Autodesk Inventor part; units mm, degrees
ref_plane "YZ Plane" through (0, 0, 0) normal (1, 0, 0) x (0, 1, 0)
ref_plane "XZ Plane" through (0, 0, 0) normal (0, 1, 0) x (-1, 0, 0)
ref_plane "XY Plane" through (0, 0, 0) normal (0, 0, 1) x (1, 0, 0)
sketch "Sketch1" plane through (0, 0, 0) normal (0, 0, 1) x (1, 0, 0)
  line L0 (0, 0) -> (25.4, 0)
  line L1 (25.4, 0) -> (25.4, 25.4)
  line L2 (25.4, 25.4) -> (0, 25.4)
  line L3 (0, 25.4) -> (0, 0)
  line L4 (1.5875, 23.8125) -> (23.8125, 23.8125)
  line L5 (23.8125, 23.8125) -> (23.8125, 1.5875)
  line L6 (23.8125, 1.5875) -> (1.5875, 1.5875)
  line L7 (1.5875, 1.5875) -> (1.5875, 23.8125)
  dimension "d0" = 25.4
  dimension "d1" = 25.4
  dimension "d4" = 1.5875
extrude "Extrusion1" add sketch "Sketch1" against normal blind 25.4 contours L3 L2 L1 L0 | L4 L5 L6 L7
extrude "Extrusion2" add sketch "Sketch1" along normal blind 25.4 contours L4 L5 L6 L7
sketch "Sketch2" plane through (25.4, 0, 0) normal (1, 0, 0) x (0, 0, -1)
  line L0 (25.4, 0) -> (25.4, 25.4)
  line L1 (0, 25.4) -> (25.4, 25.4)
  line L2 (0, 0) -> (0, 25.4)
  line L3 (0, 0) -> (25.4, 0)
  line L4 (23.8125, 23.8125) -> (23.8125, 1.5875)
  line L5 (23.8125, 1.5875) -> (1.5875, 1.5875)
  line L6 (1.5875, 1.5875) -> (1.5875, 23.8125)
  line L7 (1.5875, 23.8125) -> (23.8125, 23.8125)
  dimension "d8" = 1.5875
sketch "Sketch3" plane through (0, 25.4, 0) normal (0, 1, 0) x (1, 0, 0)
  line L0 (25.4, 25.4) -> (0, 25.4)
  line L1 (0, 0) -> (0, 25.4)
  line L2 (25.4, 0) -> (0, 0)
  line L3 (25.4, 0) -> (25.4, 25.4)
  line L4 (1.5875, 23.8125) -> (23.8125, 23.8125)
  line L5 (23.8125, 23.8125) -> (23.8125, 1.5875)
  line L6 (23.8125, 1.5875) -> (1.5875, 1.5875)
  line L7 (1.5875, 1.5875) -> (1.5875, 23.8125)
  dimension "d9" = 1.5875
extrude "Extrusion3" add sketch "Sketch2" along normal blind 25.4 contours L4 L5 L6 L7
extrude "Extrusion4" add sketch "Sketch3" along normal blind 25.4 contours L4 L5 L6 L7
sketch "Sketch4" plane through (1.5875, 25.4, -23.8125) normal (-1, 0, 0) x (0, 0, 1)
  point P0 (23.8125, -25.4)
  point P1 (11.1125, 12.7)
hole "Hole1" at (1.5875, 38.1, -12.7) direction (1, 0, 0) diameter 6.35 depth 25.4 tip angle 118
sketch "Sketch5" plane through (23.8125, 25.4, -23.8125) normal (0, 0, -1) x (-1, 0, 0)
  point P0 (23.8125, -25.4)
  point P1 (11.1125, 12.7)
hole "Hole2" at (12.7, 38.1, -23.8125) direction (0, 0, 1) diameter 6.35 depth 25.4 tip angle 118
sketch "Sketch6" plane through (1.5875, 23.8125, 25.4) normal (0, 1, 0) x (1, 0, 0)
  line L0 (0, 25.4) -> (22.225, 25.4)
  line L1 (23.8125, 25.4) -> (23.8125, 50.8)
  point P0 (-1.5875, 25.4)
  point P1 (11.1125, 12.7)
  point P2 (36.5125, 38.1)
  dimension "d28" = 12.7
  dimension "d29" = 12.7
hole "Hole3" at (12.7, 23.8125, 12.7) at (38.1, 23.8125, -12.7) direction (0, -1, 0) diameter 6.35 depth 25.4 tip angle 118
properties part number "3-way corner"
Model file for the job. Use its own axes, mm. A direction names the side the tool comes from. Coordinates: 2 decimals unless noted, no trailing zeros. Order: outer loops, then holes, each group sorted by start corner. A loop starts at its lowest first (then second) coordinate and runs counter-clockwise, first axis right, second up. Notation, with made-up numbers: M -9.75,-25 L 30.25,-25 A22 cw 30.25,-18 Z; hole C 62.5,18 d8. An arc over 180 degrees is marked long. Answer as CSV lines item,"result".
(1) Band-saw the part on C-C, the plane x = 38.1. List the corners of the cut face in (y, z) (1 decimal), then the cut area to 3 significant figures.
Geometry says:
outline,"M 1.6,-23.8 L 23.8,-23.8 L 23.8,-15.9 L 1.6,-15.9 Z; M 1.6,-9.5 L 23.8,-9.5 L 23.8,-1.6 L 1.6,-1.6 Z"
area,"353 mm2"
(2) 3-axis set-ups, long thin cutter, end or side, ignore diameter. For faces 5 (the flat face through (35, 23.812, -10)), 6 (the flat face through (1.588, 13, 13)), 7 (the flat face through (10, 23.812, 15)), 8 (the flat face through (23.812, 13, 13)): which of +Z, -Z, +X, -X, +Y, -Y reach the whole face in a straight line?
Geometry says:
face 5,"+Z, -Z, +X, +Y"
face 6,"+Z, -X, +Y, -Y"
face 7,"+Z, +X, -X, +Y"
face 8,"+Z, +X, +Y, -Y"
(3) Flat gauge pins, fed straight in: pin 1 (6.5 mm diameter, centred on x = 42.5, y = 7.5, fed in from -Z); pin 2 (12 mm diameter, centred on x = 23, y = 33, fed in from +Z); pin 3 (18 mm diameter, centred on x = 35.5, z = -9, fed in from -Y). Where does each tip first touch, or does it go through?
Geometry says:
pin 1,"stops at z = -23.81"
pin 2,"stops at z = -1.59"
pin 3,"stops at y = 1.59"
(4) Pull direction Y, two halves, no side cores. Call faces 1 (the cylindrical face through (13.92, 41.03, -19.41)), 2 (the cylindrical face through (5.987, 35.423, -10.993)), 3 (the flat face through (1.588, 35, -10)), 4 (the flat face through (13, 0, -13)): +Y half, -Y half, draft (parallel to the pull), parting line (faces both ways), or undercut.
Geometry says:
face 1,"undercut"
face 2,"undercut"
face 3,"draft"
face 4,"-Y half"
(5) Band-saw the part on D-D, the plane z = -14.5. State how many separate pieces and enclosed holes the cut face has, then the cut area to 3 significant figures.
Geometry says:
separate pieces,"3"
enclosed holes,"0"
area,"1,540 mm2"
(6) Band-saw the part on B-B, the plane z = 12.7. List the corners of the cut face in (x, y) (1 decimal).
Geometry says:
outline,"M 1.6,1.6 L 9.5,1.6 L 9.5,23.8 L 1.6,23.8 Z; M 15.9,1.6 L 23.8,1.6 L 23.8,23.8 L 15.9,23.8 Z"
(7) Wall check: line 1 along Z through (x, y) = (12.7, 8.5) (3 decimals); line 2 along Y through (x, z) = (12.7, -17.5) (3 decimals); line 3 along X through (y, z) = (38, -17). Give the ranges that are in metal, low to high.
Geometry says:
line 1,"z = -25.4 to 9.525, 15.875 to 25.4"
line 2,"y = 0 to 34.925, 41.275 to 50.8"
line 3,"x = 1.59 to 9.53, 15.87 to 23.81"
